Solid Edge part; units mm, degrees
sketch "Sketch1" plane through (0, 0, 0) normal (0, 0, 1) x (1, 0, 0)
  line L0 (93, -53) -> (93, 53)
  line L1 (93, 53) -> (-93, 53)
  line L2 (-93, 53) -> (-93, -53)
  line L3 (-93, -53) -> (93, -53)
extrude "Protrusion1" add sketch "Sketch1" along normal mid plane 2
sketch "Sketch2" plane through (0, 0, 1) normal (0, 0, 1) x (1, 0, 0)
  line L0 (-93, 53) -> (-93, -53)
  line L1 (-93, -53) -> (93, -53)
  line L2 (93, -53) -> (93, 53)
  line L3 (93, 53) -> (-93, 53)
  line L4 (-91, 51) -> (-91, -51)
  line L5 (-91, -51) -> (91, -51)
  line L6 (91, -51) -> (91, 51)
  line L7 (91, 51) -> (-91, 51)
extrude "ExtrudedProtrusion_3" add sketch "Sketch2" along normal blind 5
sketch "Sketch3" plane through (0, 0, 1) normal (0, 0, 1) x (0, 1, 0)
  circle A0 centre (45, 85) radius 4
  circle A1 centre (-45, 85) radius 4
  circle A2 centre (45, -85) radius 4
  circle A3 centre (-45, -85) radius 4
extrude "ExtrudedProtrusion_4" add sketch "Sketch3" along normal blind 3.5
hole "Hole_1" at (-85, 45, 4.5) direction (0, 0, -1) diameter 3.2 end up to next
hole "Hole_2" at (-85, -45, 4.5) direction (0, 0, -1) diameter 3.2 end up to next
hole "Hole_3" at (85, 45, 4.5) direction (0, 0, -1) diameter 3.2 end up to next
hole "Hole_4" at (85, -45, 4.5) direction (0, 0, -1) diameter 3.2 end up to next
sketch "Sketch4" plane through (0, 0, 1) normal (0, 0, 1) x (0, 1, 0)
  circle A0 centre (45, 85) radius 4
  line L0 (51, 91) -> (39, 91)
  line L1 (39, 91) -> (39, 79)
  line L2 (39, 79) -> (51, 79)
  line L3 (51, 79) -> (51, 91)
  line L4 (39, -91) -> (39, -79)
  line L5 (39, -79) -> (51, -79)
  line L6 (51, -79) -> (51, -91)
  line L7 (51, -91) -> (39, -91)
  circle A1 centre (45, -85) radius 4
  circle A2 centre (-45, -85) radius 4
  line L8 (-51, -91) -> (-39, -91)
  line L9 (-39, -91) -> (-39, -79)
  line L10 (-39, -79) -> (-51, -79)
  line L11 (-51, -79) -> (-51, -91)
  line L12 (-39, 79) -> (-51, 79)
  line L13 (-51, 79) -> (-51, 91)
  line L14 (-51, 91) -> (-39, 91)
  line L15 (-39, 91) -> (-39, 79)
  circle A3 centre (-45, 85) radius 4
extrude "Protrusion2" add sketch "Sketch4" along normal blind 2
sketch "Sketch5" plane through (0, 0, 6) normal (0, 0, 1) x (1, 0, 0)
  line L0 (91, 51) -> (-91, 51)
  line L1 (-91, 51) -> (-91, -51)
  line L2 (-91, -51) -> (91, -51)
  line L3 (91, -51) -> (91, 51)
  line L4 (-92.1, 52.1) -> (-92.1, -52.1)
  line L5 (-92.1, -52.1) -> (92.1, -52.1)
  line L6 (92.1, -52.1) -> (92.1, 52.1)
  line L7 (92.1, 52.1) -> (-92.1, 52.1)
extrude "Vyříznutí_3" cut sketch "Sketch5" against normal blind 1
fillet "Zaoblení_3" radius 1 4 edges at (93, -53, 2.5) (93, 53, 2.5) (-93, 53, 2.5) (-93, -53, 2.5)
sketch "Sketch6" plane through (0, 0, -1) normal (0, 0, -1) x (0, 1, 0)
  line L0 (48.2, -83.1525) -> (45, -81.305)
  line L1 (45, -81.305) -> (41.8, -83.1525)
  line L2 (41.8, -83.1525) -> (41.8, -86.8475)
  line L3 (41.8, -86.8475) -> (45, -88.695)
  line L4 (45, -88.695) -> (48.2, -86.8475)
  line L5 (48.2, -86.8475) -> (48.2, -83.1525)
  line L6 (-45, -81.305) -> (-41.8, -83.1525)
  line L7 (-41.8, -83.1525) -> (-41.8, -86.8475)
  line L8 (-41.8, -86.8475) -> (-45, -88.695)
  line L9 (-45, -88.695) -> (-48.2, -86.8475)
  line L10 (-48.2, -86.8475) -> (-48.2, -83.1525)
  line L11 (-48.2, -83.1525) -> (-45, -81.305)
  line L12 (-45, 81.305) -> (-41.8, 83.1525)
  line L13 (-41.8, 83.1525) -> (-41.8, 86.8475)
  line L14 (-41.8, 86.8475) -> (-45, 88.695)
  line L15 (-45, 88.695) -> (-48.2, 86.8475)
  line L16 (-48.2, 86.8475) -> (-48.2, 83.1525)
  line L17 (-48.2, 83.1525) -> (-45, 81.305)
  line L18 (45, 81.305) -> (41.8, 83.1525)
  line L19 (41.8, 83.1525) -> (41.8, 86.8475)
  line L20 (41.8, 86.8475) -> (45, 88.695)
  line L21 (45, 88.695) -> (48.2, 86.8475)
  line L22 (48.2, 86.8475) -> (48.2, 83.1525)
  line L23 (48.2, 83.1525) -> (45, 81.305)
extrude "Vyříznutí_MatkaHoles" cut sketch "Sketch6" against normal blind 2
The model under review builds one solid part; all positions refer to its coordinate system, in mm. A direction names the side the tool comes from. Round coordinates to 2 decimals unless told otherwise and drop trailing zeros. Order: outer loops, then holes, each group sorted by start corner. A loop starts at its lowest first (then second) coordinate and runs counter-clockwise, first axis right, second up. Notation, with made-up numbers: (-35, 31.25) -> (-9, 31.25) arc R27 ccw to (-9, 49.25) -> close; hole circle Ø2 at (75.25, 45.5). An arc over 180 degrees is marked (long way). Return JSON: item names as keys, results as strings.
1. Insertion check: P1, Ø7, axis at x = 85, y = 43.5, coming from the -Z side; P2, Ø10, axis at x = -7, y = -12, coming from the +Z side; P3, Ø3, axis at x = -84.5, y = -45, coming from the -Z side. Each pin has a flat end and moves straight along its axis. Give the tip position at first contact, or say it passes through.
Answer block:
{"P1": "stops at z = -1", "P2": "stops at z = 1", "P3": "stops at z = 1"}
2. The part is to be moulded in two halves that separate along Y. For faces 1 (the face through (-1, -51, 3)), 2 (the face through (93, -1, 2)), say which applies: +Y half, -Y half, draft (parallel to the pull), parting line (faces both ways), or undercut.
Answer block:
{"face 1": "undercut", "face 2": "draft"}
3. For L1, parallel to Y at x = 85, z = 2.7; L2, parallel to X at y = -45, z = 2; L3, parallel to Y at x = 85, z = 3.6, list the stretches that pass through material, from the lowest coordinate up. Write a range as [from, to].
Answer block:
{"L1": "y = [-53, -46.6], [-43.4, -39], [39, 43.4], [46.6, 53]", "L2": "x = [-93, -86.6], [-83.4, -79], [79, 83.4], [86.6, 93]", "L3": "y = [-53, -51], [-49, -46.6], [-43.4, -41], [41, 43.4], [46.6, 49], [51, 53]"}
4. For faces 3 (the face through (-83, -44, 1)), 4 (the face through (-1, 1, -1)), 5 (the face through (91, -1, 3)), list the 3-axis set-ups (+Z, -Z, +X, -X, +Y, -Y) from which the entire face can be reached by the end or side of a thin tool; tool diameter is ignored.
Answer block:
{"face 3": "-Z", "face 4": "-Z, +X, -X, +Y, -Y", "face 5": "+Z"}
5. Take a section at B-B (x = 60). Write out the cut boundary in (y, z).
Answer block:
{"outline": "(-53, -1) -> (53, -1) -> (53, 6) -> (52.1, 6) -> (52.1, 5) -> (51, 5) -> (51, 1) -> (-51, 1) -> (-51, 5) -> (-52.1, 5) -> (-52.1, 6) -> (-53, 6) -> close"}
6. Take a section at A-A (y = 23.5). Write out the cut boundary in (x, z).
Answer block:
{"outline": "(-93, -1) -> (93, -1) -> (93, 6) -> (92.1, 6) -> (92.1, 5) -> (91, 5) -> (91, 1) -> (-91, 1) -> (-91, 5) -> (-92.1, 5) -> (-92.1, 6) -> (-93, 6) -> close"}
